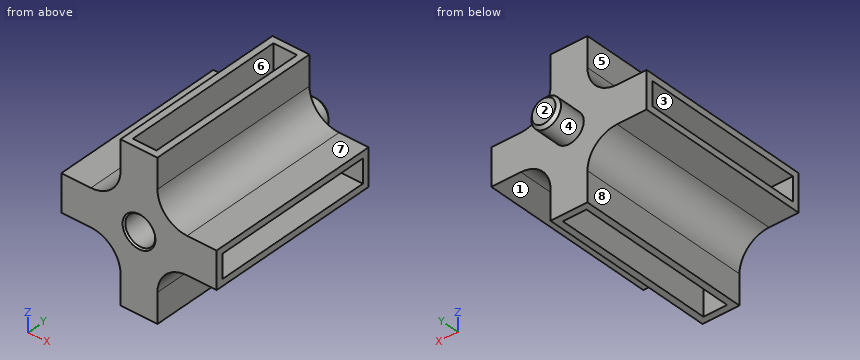
Autodesk Fusion 360 part; units mm, degrees
sketch "Sketch1" plane through (0, 0, 0) normal (0, 1, 0) x (1, 0, 0)
sketch "Sketch2" plane through (0, 0, 0) normal (0, 1, 0) x (1, 0, 0)
  line L0 (-39.0176, 15.875) -> (-15.875, 15.875)
  line L1 (-15.875, 15.875) -> (-15.875, 66.675)
  line L2 (-15.875, 66.675) -> (15.875, 66.675)
  line L3 (15.875, 66.675) -> (15.875, 15.875)
  line L4 (15.875, 15.875) -> (66.675, 15.875)
  line L5 (66.675, 15.875) -> (66.675, -15.875)
  line L6 (66.675, -15.875) -> (15.875, -15.875)
  line L7 (15.875, -15.875) -> (15.875, -66.675)
  line L8 (15.875, -66.675) -> (-15.875, -66.675)
  line L9 (-15.875, -66.675) -> (-15.875, -15.875)
  line L10 (-15.875, -15.875) -> (-66.675, -15.875)
  line L11 (-66.675, -15.875) -> (-66.675, 15.875)
  line L12 (-66.675, 15.875) -> (-39.0176, 15.875)
  line L13 (1.75, 0) -> (22.5, 0)
  line L14 (0, -1.75) -> (0, -22.5)
  dimension "d1" = 31.75
  dimension "d2" = 31.75
  dimension "d7" = 50.8
  dimension "d8" = 50.8
extrude "Extrude1" add sketch "Sketch2" along normal blind 152.4
sketch "Sketch3" plane through (-66.675, 0, 0) normal (-1, 0, 0) x (0, -1, 0)
  line L0 (0, -15.875) -> (0, 15.875)
  line L1 (0, 15.875) -> (-152.4, 15.875)
  line L2 (-152.4, 15.875) -> (-152.4, -15.875)
  line L3 (-152.4, -15.875) -> (0, -15.875)
  line L4 (-146.685, 10.16) -> (-5.715, 10.16)
  line L5 (-5.715, 10.16) -> (-5.715, -10.16)
  line L6 (-5.715, -10.16) -> (-146.685, -10.16)
  line L7 (-146.685, -10.16) -> (-146.685, 10.16)
  dimension "d11" = 140.97
  dimension "d12" = 20.32
  dimension "d13" = 5.715
  dimension "d14" = 5.715
extrude "Extrude2" cut sketch "Sketch3" against normal blind 50.8 contours L4 L5 L6 L7
mirror "Mirror1" about plane through (0, 0, 0) normal (1, 0, 0) of "Extrude2"
fillet "Fillet1" radius 25.4 1 edges at (15.875, 76.2, 15.875)
fillet "Fillet1" radius 25.4 3 edges at (-15.875, 76.2, 15.875) (-15.875, 76.2, -15.875) (15.875, 76.2, -15.875)
sketch "Sketch4" plane through (0, 0, 66.675) normal (0, 0, 1) x (-1, 0, 0)
  line L0 (15.875, 0) -> (-15.875, 0)
  line L1 (-15.875, 0) -> (-15.875, -152.4)
  line L2 (-15.875, -152.4) -> (15.875, -152.4)
  line L3 (15.875, -152.4) -> (15.875, 0)
  line L4 (10.16, -146.685) -> (-10.16, -146.685)
  line L5 (-10.16, -146.685) -> (-10.16, -5.715)
  line L6 (-10.16, -5.715) -> (10.16, -5.715)
  line L7 (10.16, -5.715) -> (10.16, -146.685)
  dimension "d24" = 5.715
  dimension "d25" = 5.715
  dimension "d26" = 5.715
  dimension "d27" = 5.715
extrude "Extrude3" cut sketch "Sketch4" against normal blind 50.8 contours L4 L5 L6 L7
mirror "Mirror2" about plane through (0, 0, 0) normal (0, 0, 1) of "Extrude3"
sketch "Sketch6" plane through (0, 152.4, 0) normal (0, 1, 0) x (-1, 0, 0)
  line L0 (66.675, -15.875) -> (66.675, 15.875)
  line L1 (66.675, 15.875) -> (41.275, 15.875)
  arc A0 (15.875, 41.275) -> (41.275, 15.875) centre (41.275, 41.275) ccw
  line L2 (15.875, 41.275) -> (15.875, 66.675)
  line L3 (15.875, 66.675) -> (-15.875, 66.675)
  line L4 (-15.875, 66.675) -> (-15.875, 41.275)
  arc A1 (-41.275, 15.875) -> (-15.875, 41.275) centre (-41.275, 41.275) ccw
  line L5 (-41.275, 15.875) -> (-66.675, 15.875)
  line L6 (-66.675, 15.875) -> (-66.675, -15.875)
  line L7 (-66.675, -15.875) -> (-41.275, -15.875)
  arc A2 (-15.875, -41.275) -> (-41.275, -15.875) centre (-41.275, -41.275) ccw
  line L8 (-15.875, -41.275) -> (-15.875, -66.675)
  line L9 (-15.875, -66.675) -> (15.875, -66.675)
  line L10 (15.875, -66.675) -> (15.875, -41.275)
  arc A3 (41.275, -15.875) -> (15.875, -41.275) centre (41.275, -41.275) ccw
  line L11 (41.275, -15.875) -> (66.675, -15.875)
  circle A4 centre (0, 0) radius 12.7
  dimension "d32" = 25.4
extrude "Extrude4" add sketch "Sketch6" along normal blind 25.4 contours A4
chamfer "Chamfer1" distance 2.54 angle 45 1 edges at (11.8406, 177.8, -4.5925)
sketch "Sketch7" plane through (0, 0, 0) normal (0, -1, 0) x (1, 0, 0)
  line L0 (-66.675, 15.875) -> (-66.675, -15.875)
  line L1 (-66.675, -15.875) -> (-41.275, -15.875)
  arc A0 (-15.875, -41.275) -> (-41.275, -15.875) centre (-41.275, -41.275) ccw
  line L2 (-15.875, -41.275) -> (-15.875, -66.675)
  line L3 (-15.875, -66.675) -> (15.875, -66.675)
  line L4 (15.875, -66.675) -> (15.875, -41.275)
  arc A1 (41.275, -15.875) -> (15.875, -41.275) centre (41.275, -41.275) ccw
  line L5 (41.275, -15.875) -> (66.675, -15.875)
  line L6 (66.675, -15.875) -> (66.675, 15.875)
  line L7 (66.675, 15.875) -> (41.275, 15.875)
  arc A2 (15.875, 41.275) -> (41.275, 15.875) centre (41.275, 41.275) ccw
  line L8 (15.875, 41.275) -> (15.875, 66.675)
  line L9 (15.875, 66.675) -> (-15.875, 66.675)
  line L10 (-15.875, 66.675) -> (-15.875, 41.275)
  arc A3 (-41.275, 15.875) -> (-15.875, 41.275) centre (-41.275, 41.275) ccw
  line L11 (-41.275, 15.875) -> (-66.675, 15.875)
  circle A4 centre (0, 0) radius 12.827
  dimension "d36" = 25.654
extrude "Extrude5" cut sketch "Sketch7" against normal blind 27.94 contours A4
chamfer "Chamfer2" distance 1.27 angle 45 1 edges at (-11.959, 0, 4.6384)
CAD build for the part. Positions are in the model's coordinates, mm. Face numbers are marked on the shaded views. A direction names the side the tool comes from. Give positions to 0.01 mm unless a question says otherwise; leave off trailing zeros. Loops run counter-clockwise (first coordinate to the right, second up) from the corner with the lowest first, then second, coordinate; pieces in that order, holes last. Notation, with made-up numbers: (79.5, 64) - (89.5, 64) arc R26 cw to (89.5, 86) - close; hole circle Ø5 at (70.25, 47). An arc over 180 degrees is marked (long way). Put each result on its own line as item: value.
Q1. Slice it at D-D (x = 51). Give the cut face in (y, z) (3 decimals).
Filled in:
outline: (0, -15.875) - (152.4, -15.875) - (152.4, 15.875) - (0, 15.875) - close; hole (5.715, -10.16) - (146.685, -10.16) - (146.685, 10.16) - (5.715, 10.16) - close
Q2. Flat gauge pins, fed straight in: pin 1 (1.5 mm diameter, centred on x = 39.5, y = 103, fed in from -Z); pin 2 (2 mm diameter, centred on y = 106.5, z = 26, fed in from -X); pin 3 (12.5 mm diameter, centred on y = 89, z = -53.5, fed in from +X) (3 decimals). Where does each tip first touch, or does it go through?
Filled in:
pin 1: stops at z = -16
pin 2: stops at x = -21.77
pin 3: stops at x = 15.875
Q3. Mould opens along Y. For the marked faces 1, 2 and 3 say: pulls with the +Y half, pulls with the -Y half, needs draft (parallel to the pull), parting line crosses it, or undercut.
Filled in:
face 1: needs draft
face 2: pulls with the +Y half
face 3: undercut
Q4. Slice it at A-A (x = 0). Give the cut face in (y, z) (3 decimals), plus the area to 3 significant figures.
Filled in:
outline: (0, -66.675) - (5.715, -66.675) - (5.715, -15.875) - (146.685, -15.875) - (146.685, -66.675) - (152.4, -66.675) - (152.4, -12.7) - (175.26, -12.7) - (177.8, -10.16) - (177.8, 10.16) - (175.26, 12.7) - (152.4, 12.7) - (152.4, 66.675) - (146.685, 66.675) - (146.685, 15.875) - (5.715, 15.875) - (5.715, 66.675) - (0, 66.675) - (0, 14.097) - (1.27, 12.827) - (27.94, 12.827) - (27.94, -12.827) - (1.27, -12.827) - (0, -14.097) - close
area: 5,920 mm²
Q5. Tool access for the marked faces 4, 5, 6, 7 and 8: list every direction of +Z, -Z, +X, -X, +Y, -Y with a clear straight run to the whole face (end or side of a thin tool).
Filled in:
face 4: +Y
face 5: +Z, -X, +Y, -Y
face 6: +Z
face 7: +Z, +X, +Y, -Y
face 8: -Z, -X, +Y, -Y
Q6. Slice it at C-C (z = -28.5). Give the cut face in (x, y) (3 decimals), plus the area to 3 significant figures.
Filled in:
outline: (-19.321, 0) - (19.321, 0) - (19.321, 152.4) - (-19.321, 152.4) - close; hole (-10.16, 5.715) - (10.16, 5.715) - (10.16, 146.685) - (-10.16, 146.685) - close
area: 3,020 mm²
Q7. Probe line 1 along Y through (x, z) = (-7.5, -56) (3 decimals); line 2 along Z through (x, y) = (0, 17) (3 decimals); line 3 along X through (y, z) = (71, -44) (3 decimals). List the from-to ranges inside material, lowest first.
Filled in:
line 1: y = 0 to 5.715, 146.685 to 152.4
line 2: z = -15.875 to -12.827, 12.827 to 15.875
line 3: x = -15.875 to -10.16, 10.16 to 15.875
